from build123d import *

# Parameters (mm, degrees)
SKETCH1_R               = 6.35
SKETCH1_R_2             = 5.461
EXTRUDE1_DEPTH          = 114.3
SKETCH2_R               = 2
CUT_EXTRUDE1_DEPTH      = 38.1
CUT_EXTRUDE1_DEPTH_BACK = 38.1


with BuildPart() as part:
    # Sketch1 → Extrude1 (new body)
    with BuildSketch(Plane.XY):
        Circle(SKETCH1_R)
        Circle(SKETCH1_R_2, mode=Mode.SUBTRACT)
    extrude(amount=EXTRUDE1_DEPTH)

    # Sketch2 → Cut-Extrude1 (cut, two sides)
    with BuildSketch(Plane(origin=(0, 0, 0), x_dir=(1, 0, 0), z_dir=(0, 1, 0))) as cut_extrude1_sk:
        with Locations(Location((0, -9.525, 0), (0, 0, 270))):  # turned: the seam where the file's is
            Circle(SKETCH2_R)
        with Locations(Location((0, -104.775, 0), (0, 0, 270))):  # turned: the seam where the file's is
            Circle(SKETCH2_R)
    extrude(amount=CUT_EXTRUDE1_DEPTH, mode=Mode.SUBTRACT)
    extrude(cut_extrude1_sk.sketch, amount=-CUT_EXTRUDE1_DEPTH_BACK, mode=Mode.SUBTRACT)


solid = part.part
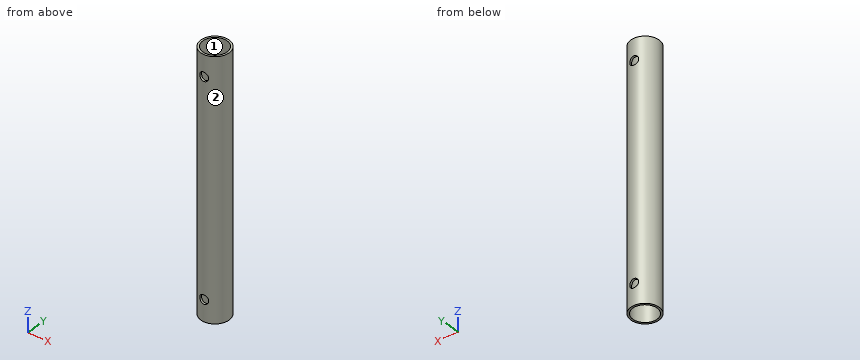
Could you check a few things on this model? Use its own coordinates, in mm. Face numbers are marked on the shaded views. Coordinates: 2 decimals unless noted, no trailing zeros. Order: outer loops, then holes, each group sorted by start corner. A loop starts at its lowest first (then second) coordinate and runs counter-clockwise, first axis right, second up.
Q1. Thinking about a two-plate mould opening in Y: for the marked faces 1 and 2, which applies, released by +Y, released by -Y, zero draft, split by the parting line, or undercut?
Q2. Please list where these lines run through material, in increasing order: L1, parallel to Z at x = 0, y = -5.95 (3 decimals); L2, parallel to Y at x = 0, z = 72; L3, parallel to Y at x = -4, z = 98.
Q3. Suppose I cut it at B-B on x = -3.25. Please give me the cut outline in (y, z).
Q4. Suppose I cut it at A-A on y = 0. Please give me the cut outline in (x, z), and give its area (3 significant figures).
Q5. Will these pins go through, and if not, where does the flat tip stop? pin 1 (2 mm diameter, centred on x = -4, z = 61.5, fed in from -Y); pin 2 (2 mm diameter, centred on y = 1.5, z = 68.5, fed in from +X); pin 3 (2 mm diameter, centred on x = 3, z = 67.5, fed in from +Y).
Q6. Suppose I cut it at C-C on z = 35. Please give me the cut outline in (x, y), and give its area (3 significant figures).
Answer:
1. face 1: undercut
1. face 2: split by the parting line
2. L1: z = 0 to 7.525, 11.525 to 102.775, 106.775 to 114.3
2. L2: y = -6.35 to -5.46, 5.46 to 6.35
2. L3: y = -4.93 to -3.72, 3.72 to 4.93
3. outline: (-5.46, 0) - (-4.39, 0) - (-4.39, 114.3) - (-5.46, 114.3) - close; (4.39, 0) - (5.46, 0) - (5.46, 114.3) - (4.39, 114.3) - close
4. outline: (-6.35, 0) - (-5.46, 0) - (-5.46, 114.3) - (-6.35, 114.3) - close; (5.46, 0) - (6.35, 0) - (6.35, 114.3) - (5.46, 114.3) - close
4. area: 203 mm2
5. pin 1: stops at y = -5.6
5. pin 2: stops at x = 6.33
5. pin 3: stops at y = 6.03
6. outline: circle Ø12.7 at (0, 0); hole circle Ø10.92 at (0, 0)
6. area: 33.0 mm2
